from build123d import *

# Parameters (mm, degrees)
BOSS_EXTRUDE1_DEPTH = 5
SKETCH2_R           = 1.5
CUT_EXTRUDE1_DEPTH  = 10


with BuildPart() as part:
    # Sketch1 → Boss-Extrude1 (new, symmetric)
    with BuildSketch(Plane.XY):
        with BuildLine():
            Line((-7.167342336, 1.25), (-7.167342336, 2.45))
            Line((-7.167342336, 2.45), (-2.167342336, 2.45))
            ThreePointArc((-2.167342336, 2.45), (3.271066004, 0), (-2.167342336, -2.45))
            Line((-2.167342336, -2.45), (-7.167342336, -2.45))
            Line((-7.167342336, -2.45), (-7.167342336, -1.25))
            Line((-7.167342336, -1.25), (-2.167342336, -1.25))
            Line((-2.167342336, -1.25), (-2.167342336, -1.246044622))
            ThreePointArc((-2.167342336, -1.246044622), (2.5, 0), (-2.167342336, 1.246044622))
            Line((-2.167342336, 1.246044622), (-2.167342336, 1.25))
            Line((-2.167342336, 1.25), (-7.167342336, 1.25))
        make_face()
    extrude(amount=BOSS_EXTRUDE1_DEPTH, both=True)

    # Sketch2 → Cut-Extrude1 (cut)
    with BuildSketch(Plane(origin=(0, 2.45, 0), x_dir=(1, 0, 0), z_dir=(0, 1, 0))):
        with Locations(Location((-4.667342336, 0, 0), (0, 0, 180))):
            Circle(SKETCH2_R)
    extrude(amount=-CUT_EXTRUDE1_DEPTH, mode=Mode.SUBTRACT)


solid = part.part
Geometry check sheet. Reference: the model listing, model coordinates, mm. A direction names the side the tool comes from. Round coordinates to 2 decimals unless told otherwise and drop trailing zeros. Order: outer loops, then holes, each group sorted by start corner. A loop starts at its lowest first (then second) coordinate and runs counter-clockwise, first axis right, second up. Notation, with made-up numbers: M 52.5,47 L 69.5,47 A16 cw 69.5,77 Z; hole C 62,74 d6. An arc over 180 degrees is marked long. Write each question's results on one line, items separated by ' | '. Start each with the question number.
1. Cross-section at A-A on x = 0. Record the boundary of the cut face in (y, z).
2. Cross-section at B-B on y = -2. Record the boundary of the cut face in (x, z).
3. Set-up check for faces 4 (the face through (-3.5, -2.45, 1.2)), 5 (the face through (-6.1, -1.84, 0.45)), 6 (the face through (-6, 2.45, 1)), 7 (the face through (-3.5, 1.25, 1.2)), 8 (the face through (-2.3, 1.5, -5)): record each of +Z, -Z, +X, -X, +Y, -Y from which the full face is reachable in a straight line by a thin tool's end or side.
4. Go/stop test with flat-tipped pins: P1, Ø5.5, axis at x = -5, z = 2, coming from the +Y side; P2, Ø1.5, axis at x = -5, z = -1.5, coming from the -Y side; P3, Ø3, axis at y = -2.5, z = 2.5, coming from the +X side. Record where each tip stops, or that it passes through.
5. Cross-section at C-C on x = -5. Record the boundary of the cut face in (y, z).
6. Draft check along X on faces 1 (the face through (-2.3, 1.5, 5)), 2 (the face through (-7.167, 2, 0)), 3 (the face through (2.5, -0.1, 0.1)). Enter one of: pulls with the +X half, pulls with the -X half, needs draft (parallel to the pull), parting line crosses it, or undercut.
7. Material ranges on L1, parallel to Y at x = -3.5, z = 1; L2, parallel to Y at x = -1.25, z = 4.5; L3, parallel to X at y = -2, z = -3.5, recorded low to high. Write a range as from..to.
Resolved:
1) outline: M -3.27,-5 L -2.5,-5 L -2.5,5 L -3.27,5 Z; M 2.5,-5 L 3.27,-5 L 3.27,5 L 2.5,5 Z
2) outline: M -7.17,-5 L -1.5,-5 L -1.5,5 L -7.17,5 Z; M 1.5,-5 L 2.59,-5 L 2.59,5 L 1.5,5 Z; hole C -4.67,0 d3
3) face 4: +Z, -Z, -X, -Y | face 5: +Y, -Y | face 6: +Z, -Z, -X, +Y | face 7: +Z, -Z, -X | face 8: -Z, +X, -X, +Y, -Y
4) P1: y = 2.45 | P2: y = -2.45 | P3: x = 3.11
5) outline: M -2.45,-5 L -1.25,-5 L -1.25,-1.46 L -2.45,-1.46 Z; M -2.45,1.46 L -1.25,1.46 L -1.25,5 L -2.45,5 Z; M 1.25,-5 L 2.45,-5 L 2.45,-1.46 L 1.25,-1.46 Z; M 1.25,1.46 L 2.45,1.46 L 2.45,5 L 1.25,5 Z
6) face 1: needs draft | face 2: pulls with the -X half | face 3: undercut
7) L1: -2.45..-1.25, 1.25..2.45 | L2: -3.02..-2.17, 2.17..3.02 | L3: -7.17..-1.5, 1.5..2.59
